from build123d import *

# Parameters (mm, degrees)
F1_DEPTH = 10
F2_R     = 5
F3_T     = -2


with BuildPart() as f1:
    # F0 (on Top) → F1 (new body)
    with BuildSketch(Plane.XY):
        Polygon((-27.30897, 22.857411), (-31.732832, -1.598505), (-17.568031, -22.019591), (6.887884, -26.443453), (27.30897, -12.278652), (31.732832, 12.177263), (17.568031, 32.59835), (-6.887884, 37.022211), align=None)
    extrude(amount=F1_DEPTH)

    # F2
    f2_edges = [f1.edges().sort_by_distance(p)[0] for p in [
        (-5.340074, -24.231522, 10),
        (17.098427, -19.361053, 10),
        (29.520901, -0.050694, 10),
        (24.650432, 22.387806, 10),
        (5.340074, 34.810281, 10),
        (-17.098427, 29.939811, 10),
        (-29.520901, 10.629453, 10),
        (-24.650432, -11.809048, 10),
    ]]
    fillet(f2_edges, radius=F2_R)

    # F3
    f3_openings = [f1.faces().sort_by_distance(p)[0] for p in [
        (0, 5.289379, 0),
    ]]
    offset(amount=F3_T, openings=f3_openings)


solid = f1.part
Could you check a few things on this model? Use its own coordinates, in mm. A direction names the side the tool comes from. Give positions to 0.01 mm unless a question says otherwise; leave off trailing zeros. Order: outer loops, then holes, each group sorted by start corner. A loop starts at its lowest first (then second) coordinate and runs counter-clockwise, first axis right, second up.
1. For faces 1 (the cylindrical face through (-22.21, -10.31, 7.1)), 2 (the cylindrical face through (28.149, 0.374, 8.496)), which set-ups out of +Z, -Z, +X, -X, +Y, -Y let a thin tool reach every point of the face, with its end or its side?
2. I need wall thicknesses on L1, parallel to Z at x = -3.5, y = -15.5; L2, parallel to X at y = -8, z = 2.5; L3, parallel to X at y = 0, z = 6.75. Which ranges of each line are inside material? Lowest first, please.
3. Will these pins go through, and if not, where does the flat tip stop? P1, Ø6, axis at x = 18.5, y = -7.5, coming from the -Z side; P2, Ø4, axis at x = -12, z = 3, coming from the -Y side; P3, Ø2, axis at y = 22, z = 6, coming from the -X side.
4. We'd pull the mould along X, two halves only. Please class faces 3 (the flat face through (-15.825, 28.389, 2.465)), 4 (the flat face through (-24.75, -11.666, 2.465)), 5 (the flat face through (24.75, 22.245, 2.465)): pulls with the +X half, pulls with the -X half, needs draft (parallel to the pull), parting line crosses it, or undercut.
5. Suppose I cut it at B-B (z = 9). List the corners of the cut face in (x, y) for me, plus the area to 3 significant figures.
6. Suppose I cut it at A-A (z = 2). List the corners of the cut face in (x, y) for me.
Solved:
1. face 1: -Z
1. face 2: +Z, +X, -Y
2. L1: z = 8 to 10
2. L2: x = -27.29 to -24.86, 26.05 to 28.08
2. L3: x = -31.12 to -28.84, 26.93 to 29.21
3. P1: stops at z = 8
3. P2: stops at y = -23.39
3. P3: stops at x = -27.6
4. face 3: undercut
4. face 4: pulls with the -X half
4. face 5: pulls with the +X half
5. outline: (-29.62, -1.14) - (-16.4, -20.2) - (6.43, -24.33) - (25.49, -11.11) - (29.62, 11.72) - (16.4, 30.78) - (-6.43, 34.91) - (-25.49, 21.69) - close
5. area: 2,600 mm2
6. outline: (-31.73, -1.6) - (-17.57, -22.02) - (6.89, -26.44) - (27.31, -12.28) - (31.73, 12.18) - (17.57, 32.6) - (-6.89, 37.02) - (-27.31, 22.86) - close; hole (-29.62, -1.14) - (-16.4, -20.2) - (6.43, -24.33) - (25.49, -11.11) - (29.62, 11.72) - (16.4, 30.78) - (-6.43, 34.91) - (-25.49, 21.69) - close
